Read the model definition and answer for the solid it produces. Units are mm, in the model's axes. Face numbers are marked on the shaded views. A direction names the side the tool comes from. Coordinates: 2 decimals unless noted, no trailing zeros. Order: outer loops, then holes, each group sorted by start corner. A loop starts at its lowest first (then second) coordinate and runs counter-clockwise, first axis right, second up.
from build123d import *

# Parameters (mm, degrees)
F0_R      = 2.5
F1_DEPTH  = 17
F3_DEPTH  = 5
F4_W      = 46
F4_H      = 17
F5_DEPTH  = 2
F7_DEPTH  = 5
F9_W      = 13
F9_H      = 22
F10_DEPTH = 20
F11_W     = 37
F11_H     = 37
F11_R     = 2
F11_W_2   = 13
F11_H_2   = 22
F12_DEPTH = 5
F13_W     = 9
F13_H     = 19
F14_DEPTH = 10
F15_W     = 6
F15_H     = 18
F16_DEPTH = 10
F8_W      = 17
F8_H      = 30
F8_W_2    = 2
F8_H_2    = 17.5
F17_DEPTH = 5
F18_W     = 37
F18_H     = 37
F18_R     = 2
F19_DEPTH = 5
F20_DEPTH = 75.001


with BuildPart() as f1:
    # F0 (on Front) → F1 (new body)
    with BuildSketch(Plane.XZ):
        with BuildLine():
            Line((-22.4465147161, -20), (22.5534852839, -20))
            ThreePointArc((22.5534852839, -20), (26.0890191899, -18.5355339059), (27.5534852839, -15))
            Line((27.5534852839, -15), (27.5534852839, 15))
            ThreePointArc((27.5534852839, 15), (26.0890191899, 18.5355339059), (22.5534852839, 20))
            Line((22.5534852839, 20), (-22.4465147161, 20))
            ThreePointArc((-22.4465147161, 20), (-25.982048622, 18.5355339059), (-27.4465147161, 15))
            Line((-27.4465147161, 15), (-27.4465147161, -15))
            ThreePointArc((-27.4465147161, -15), (-25.982048622, -18.5355339059), (-22.4465147161, -20))
        make_face()
        with Locations((-17.4465147161, -15)):
            Circle(F0_R, mode=Mode.SUBTRACT)
        with Locations((0.0534852839, -15)):
            Circle(F0_R, mode=Mode.SUBTRACT)
        with Locations((17.5534852839, -15)):
            Circle(F0_R, mode=Mode.SUBTRACT)
        with Locations((-17.4465147161, 15)):
            Circle(F0_R, mode=Mode.SUBTRACT)
        with Locations((0.0534852839, 15)):
            Circle(F0_R, mode=Mode.SUBTRACT)
        with Locations((17.5534852839, 15)):
            Circle(F0_R, mode=Mode.SUBTRACT)
    extrude(amount=F1_DEPTH)

    # F2 (on face) → F3 (cut)
    with BuildSketch(Plane.XZ.offset(17)):
        with BuildLine():
            Line((22, 9.5), (-22, 9.5))
            ThreePointArc((-22, 9.5), (-22.7071067812, 9.2071067812), (-23, 8.5))
            Line((-23, 8.5), (-23, -8.5))
            ThreePointArc((-23, -8.5), (-22.7071067812, -9.2071067812), (-22, -9.5))
            Line((-22, -9.5), (22, -9.5))
            ThreePointArc((22, -9.5), (22.7071067812, -9.2071067812), (23, -8.5))
            Line((23, -8.5), (23, 8.5))
            ThreePointArc((23, 8.5), (22.7071067812, 9.2071067812), (22, 9.5))
        make_face()
    extrude(amount=-F3_DEPTH, mode=Mode.SUBTRACT)

    # F4 (on face) → F5 (cut)
    with BuildSketch(Plane.XZ.offset(12)):
        Rectangle(F4_W, F4_H)
    extrude(amount=-F5_DEPTH, mode=Mode.SUBTRACT)

    # F6 (on face) → F7 (cut)
    with BuildSketch(Plane.XZ.offset(10)):
        with BuildLine():
            ThreePointArc((-20.25, 7.5), (-20.7803300859, 7.2803300859), (-21, 6.75))
            Line((-21, 6.75), (-21, -6.75))
            ThreePointArc((-21, -6.75), (-20.7803300859, -7.2803300859), (-20.25, -7.5))
            ThreePointArc((-20.25, -7.5), (-19.7196699141, -7.2803300859), (-19.5, -6.75))
            Line((-19.5, -6.75), (-19.5, 6.75))
            ThreePointArc((-19.5, 6.75), (-19.7196699141, 7.2803300859), (-20.25, 7.5))
        make_face()
        with BuildLine():
            ThreePointArc((-15.75, 7.5), (-16.2803300859, 7.2803300859), (-16.5, 6.75))
            Line((-16.5, 6.75), (-16.5, -6.75))
            ThreePointArc((-16.5, -6.75), (-16.2803300859, -7.2803300859), (-15.75, -7.5))
            ThreePointArc((-15.75, -7.5), (-15.2196699141, -7.2803300859), (-15, -6.75))
            Line((-15, -6.75), (-15, 6.75))
            ThreePointArc((-15, 6.75), (-15.2196699141, 7.2803300859), (-15.75, 7.5))
        make_face()
        with BuildLine():
            ThreePointArc((-11.25, 7.5), (-11.7803300859, 7.2803300859), (-12, 6.75))
            Line((-12, 6.75), (-12, -6.75))
            ThreePointArc((-12, -6.75), (-11.7803300859, -7.2803300859), (-11.25, -7.5))
            ThreePointArc((-11.25, -7.5), (-10.7196699141, -7.2803300859), (-10.5, -6.75))
            Line((-10.5, -6.75), (-10.5, 6.75))
            ThreePointArc((-10.5, 6.75), (-10.7196699141, 7.2803300859), (-11.25, 7.5))
        make_face()
        with BuildLine():
            ThreePointArc((-6.75, 7.5), (-7.2803300859, 7.2803300859), (-7.5, 6.75))
            Line((-7.5, 6.75), (-7.5, -6.75))
            ThreePointArc((-7.5, -6.75), (-7.2803300859, -7.2803300859), (-6.75, -7.5))
            ThreePointArc((-6.75, -7.5), (-6.2196699141, -7.2803300859), (-6, -6.75))
            Line((-6, -6.75), (-6, 6.75))
            ThreePointArc((-6, 6.75), (-6.2196699141, 7.2803300859), (-6.75, 7.5))
        make_face()
        with BuildLine():
            ThreePointArc((-2.25, 7.5), (-2.7803300859, 7.2803300859), (-3, 6.75))
            Line((-3, 6.75), (-3, -6.75))
            ThreePointArc((-3, -6.75), (-2.7803300859, -7.2803300859), (-2.25, -7.5))
            ThreePointArc((-2.25, -7.5), (-1.7196699141, -7.2803300859), (-1.5, -6.75))
            Line((-1.5, -6.75), (-1.5, 6.75))
            ThreePointArc((-1.5, 6.75), (-1.7196699141, 7.2803300859), (-2.25, 7.5))
        make_face()
        with BuildLine():
            ThreePointArc((2.25, 7.5), (1.7196699141, 7.2803300859), (1.5, 6.75))
            Line((1.5, 6.75), (1.5, -6.75))
            ThreePointArc((1.5, -6.75), (1.7196699141, -7.2803300859), (2.25, -7.5))
            ThreePointArc((2.25, -7.5), (2.7803300859, -7.2803300859), (3, -6.75))
            Line((3, -6.75), (3, 6.75))
            ThreePointArc((3, 6.75), (2.7803300859, 7.2803300859), (2.25, 7.5))
        make_face()
        with BuildLine():
            ThreePointArc((6.75, 7.5), (6.2196699141, 7.2803300859), (6, 6.75))
            Line((6, 6.75), (6, -6.75))
            ThreePointArc((6, -6.75), (6.2196699141, -7.2803300859), (6.75, -7.5))
            ThreePointArc((6.75, -7.5), (7.2803300859, -7.2803300859), (7.5, -6.75))
            Line((7.5, -6.75), (7.5, 6.75))
            ThreePointArc((7.5, 6.75), (7.2803300859, 7.2803300859), (6.75, 7.5))
        make_face()
        with BuildLine():
            ThreePointArc((11.25, 7.5), (10.7196699141, 7.2803300859), (10.5, 6.75))
            Line((10.5, 6.75), (10.5, -6.75))
            ThreePointArc((10.5, -6.75), (10.7196699141, -7.2803300859), (11.25, -7.5))
            ThreePointArc((11.25, -7.5), (11.7803300859, -7.2803300859), (12, -6.75))
            Line((12, -6.75), (12, 6.75))
            ThreePointArc((12, 6.75), (11.7803300859, 7.2803300859), (11.25, 7.5))
        make_face()
        with BuildLine():
            ThreePointArc((15.75, 7.5), (15.2196699141, 7.2803300859), (15, 6.75))
            Line((15, 6.75), (15, -6.75))
            ThreePointArc((15, -6.75), (15.2196699141, -7.2803300859), (15.75, -7.5))
            ThreePointArc((15.75, -7.5), (16.2803300859, -7.2803300859), (16.5, -6.75))
            Line((16.5, -6.75), (16.5, 6.75))
            ThreePointArc((16.5, 6.75), (16.2803300859, 7.2803300859), (15.75, 7.5))
        make_face()
        with BuildLine():
            ThreePointArc((20.25, 7.5), (19.7196699141, 7.2803300859), (19.5, 6.75))
            Line((19.5, 6.75), (19.5, -6.75))
            ThreePointArc((19.5, -6.75), (19.7196699141, -7.2803300859), (20.25, -7.5))
            ThreePointArc((20.25, -7.5), (20.7803300859, -7.2803300859), (21, -6.75))
            Line((21, -6.75), (21, 6.75))
            ThreePointArc((21, 6.75), (20.7803300859, 7.2803300859), (20.25, 7.5))
        make_face()
    extrude(amount=-F7_DEPTH, mode=Mode.SUBTRACT)

    # F9 (on face) → F10 (join)
    with BuildSketch(Plane.YZ.offset(27.5534852839)):
        with Locations((-10.5, 0)):
            Rectangle(F9_W, F9_H)
    extrude(amount=F10_DEPTH)

    # F11 (on face) → F12 (join)
    with BuildSketch(Plane.YZ.offset(47.5534852839)):
        with Locations((-11, 0)):
            Rectangle(F11_W, F11_H)
        with Locations((-24.5, -13)):
            Circle(F11_R, mode=Mode.SUBTRACT)
        with Locations((2.5, -13)):
            Circle(F11_R, mode=Mode.SUBTRACT)
        with Locations((-24.5, 13)):
            Circle(F11_R, mode=Mode.SUBTRACT)
        with Locations((-10.5, 0)):
            Rectangle(F11_W_2, F11_H_2, mode=Mode.SUBTRACT)
        with Locations((2.5, 13)):
            Circle(F11_R, mode=Mode.SUBTRACT)
    extrude(amount=-F12_DEPTH)

    # F13 (on face) → F14 (cut)
    with BuildSketch(Plane.YZ.offset(47.5534852839)):
        with Locations((-11, 0)):
            Rectangle(F13_W, F13_H)
    extrude(amount=-F14_DEPTH, mode=Mode.SUBTRACT)

    # F15 (on face) → F16 (cut)
    with BuildSketch(Plane.YZ.offset(37.5534852839)):
        with Locations((-11, 0)):
            Rectangle(F15_W, F15_H)
    extrude(amount=-F16_DEPTH, mode=Mode.SUBTRACT)

    # F8 (on face) → F17 (join)
    with BuildSketch(Plane(origin=(-27.4465147161, 0, 0), x_dir=(0, -1, 0), z_dir=(-1, 0, 0))):
        with Locations((8.5, 0)):
            Rectangle(F8_W, F8_H)
        with Locations((11, 0.25)):
            Rectangle(F8_W_2, F8_H_2, mode=Mode.SUBTRACT)
    extrude(amount=F17_DEPTH)

    # F18 (on face) → F19 (join)
    with BuildSketch(Plane(origin=(-32.4465147161, 0, 0), x_dir=(0, -1, 0), z_dir=(-1, 0, 0))):
        with Locations((11.0123828505, 0.0414154201)):
            Rectangle(F18_W, F18_H)
        with Locations((-2.4876171495, -12.9585845799)):
            Circle(F18_R, mode=Mode.SUBTRACT)
        with Locations((24.5123828505, -12.9585845799)):
            Circle(F18_R, mode=Mode.SUBTRACT)
        with Locations((-2.4876171495, 13.0414154201)):
            Circle(F18_R, mode=Mode.SUBTRACT)
        with Locations((24.5123828505, 13.0414154201)):
            Circle(F18_R, mode=Mode.SUBTRACT)
    extrude(amount=F19_DEPTH)

    # F8 (on face) → F20 (cut, through all)
    with BuildSketch(Plane(origin=(-27.4465147161, 0, 0), x_dir=(0, -1, 0), z_dir=(-1, 0, 0))):
        with Locations((11, 0.25)):
            Rectangle(F8_W_2, F8_H_2)
    extrude(amount=-F20_DEPTH, mode=Mode.SUBTRACT)


solid = f1.part
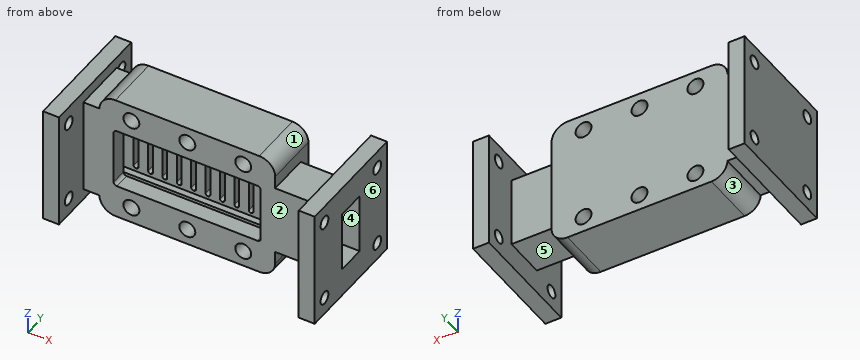
Q1. The part is cut by section A-A, the plane y = -19. Determine the outline of the cut face in (x, z), then the cut area to 3 significant figures.
Q2. Straight lines are drawn through the part: L1, parallel to Z at x = 45.3, y = -24.5; L2, parallel to X at y = -18.5, z = -14.5; L3, parallel to Z at x = 21, y = -16.5. For each, find the intervals that lie inside material, in ascending order.
Q3. Which of the six approach directions +Z, -Z, +X, -X, +Y, -Y give full straight-line access (tool end or side, diameter ignored) to the marked faces 1, 2 and 3?
Q4. Determine the mould class of the marked faces 4, 5 and 6 for opening direction Z: +Z half, -Z half, draft (parallel to the pull), parting line (faces both ways), or undercut.
Q5. The part is cut by section B-B, the plane x = -31. Determine the outline of the cut face in (y, z), then the cut area to 3 significant figures.
Q6. Each of these flat-tipped pins is pushed along its axis until it touches: P1, Ø5.5, axis at y = -8.5, z = -2.5, coming from the +X side; P2, Ø10.5, axis at x = 37, y = -11, coming from the -Z side; P3, Ø0.8, axis at x = -2, z = 1.5, coming from the -Y side; P4, Ø12, axis at x = -16, z = 8, coming from the +Y side. Where does it stop, or does it pass through?
Q7. The part is cut by section C-C, the plane x = 24. Determine the outline of the cut face in (y, z), then the cut area to 3 significant figures.
Computed values:
1. outline: (-37.45, -18.46) - (-32.45, -18.46) - (-32.45, 18.54) - (-37.45, 18.54) - close; (42.55, -18.5) - (47.55, -18.5) - (47.55, 18.5) - (42.55, 18.5) - close
1. area: 370 mm2
2. L1: z = -18.5 to -15, -11 to 11, 15 to 18.5
2. L2: x = -37.45 to -32.45, 42.55 to 47.55
2. L3: z = -20 to -9.5, 9.5 to 20
3. face 1: +Z, +Y, -Y
3. face 2: +Z, -Z, -Y
3. face 3: -Z, +Y, -Y
4. face 4: undercut
4. face 5: -Z half
4. face 6: draft
5. outline: (-17, -15) - (0, -15) - (0, 15) - (-17, 15) - close; hole (-12, -8.5) - (-10, -8.5) - (-10, 9) - (-12, 9) - close
5. area: 475 mm2
6. P1: stops at x = 47.55
6. P2: stops at z = -11
6. P3: stops at y = -5
6. P4: stops at y = 0
7. outline: (-17, -19.79) - (0, -19.79) - (0, 19.79) - (-17, 19.79) - close; hole (-12, -8.5) - (-10, -8.5) - (-10, 9) - (-12, 9) - close
7. area: 638 mm2
